Geometry check sheet. Reference: the model listing, model coordinates, mm. Face numbers are marked on the shaded views. A direction names the side the tool comes from. Give positions to 0.01 mm unless a question says otherwise; leave off trailing zeros. Loops run counter-clockwise (first coordinate to the right, second up) from the corner with the lowest first, then second, coordinate; pieces in that order, holes last. Notation, with made-up numbers: (9.25, -38) - (33.25, -38) arc R24 ccw to (33.25, 0) - close; hole circle Ø9 at (-2.5, -36.5). An arc over 180 degrees is marked (long way). Use a Markdown table: item, result. Add a question column.
1. Cross-section at C-C on y = 8.75. Enter the section's corners in (x, z), and give its area (3 significant figures).
2. Draft check along Z on the marked faces 1, 2 and 3. Enter one of: pulls with the +Z half, pulls with the -Z half, needs draft (parallel to the pull), parting line crosses it, or undercut.
3. Set-up check for the marked faces 4, 5, 6, 7 and 8: record each of +Z, -Z, +X, -X, +Y, -Y from which the full face is reachable in a straight line by a thin tool's end or side.
4. Cross-section at B-B on z = 6. Enter the section's corners in (x, y), and give its area (3 significant figures).
5. Cross-section at D-D on x = 15. Enter the section's corners in (y, z).
6. Material ranges on L1, parallel to X at y = 3.65, z = 6; L2, parallel to Z at x = -15, y = 3.85; L3, parallel to X at y = 8.75, z = 8, recorded low to high.
7. Depth check by flat-ended pin: P1, Ø2, axis at y = 7, z = 9, coming from the -X side; P2, Ø3.5, axis at x = 17.5, z = 9, coming from the +Y side; P3, Ø5, axis at x = -1, z = 4.5, coming from the -Y side. Enter the tip coordinate at first touch or a pass-through.
8. Cross-section at A-A on y = 2.75. Enter the section's corners in (x, z).
from build123d import *

# Parameters (mm, degrees)
EXTRUDE_1_DEPTH     = 12
SKETCH_2_R          = 1.9
CUT_EXTRUDE_5_DEPTH = 30.966648128


with BuildPart() as part:
    # 草图1 → 凸台-拉伸1 (new body)
    with BuildSketch(Plane.XY):
        Polygon((-11, 15), (11, 15), (11, 5), (23, 5), (23, 0), (6, 0), (6, 10), (-6, 10), (-6, 0), (-23, 0), (-23, 5), (-11, 5), align=None)
    extrude(amount=EXTRUDE_1_DEPTH)

    # 草图2 → 切除-拉伸5 (cut, through all)
    with BuildSketch(Plane(origin=(0, 0, 0), x_dir=(1, 0, 0), z_dir=(0, 1, 0))):
        with Locations((-15, -6)):
            Circle(SKETCH_2_R)
        with Locations(Location((15, -6, 0), (0, 0, 90))):
            Circle(SKETCH_2_R)
    extrude(amount=CUT_EXTRUDE_5_DEPTH, mode=Mode.SUBTRACT)


solid = part.part
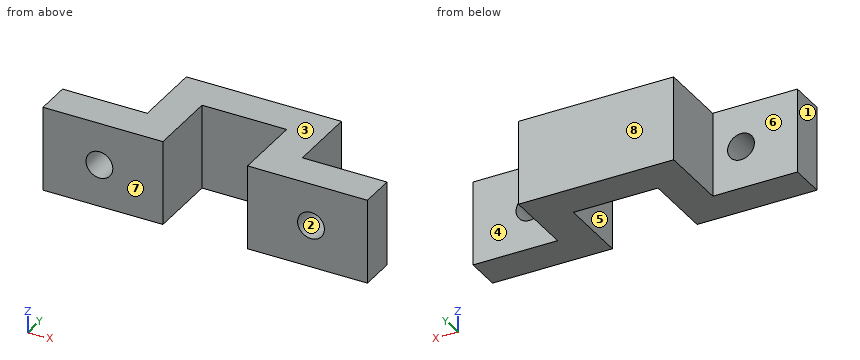
Values found:
| question | item | result |
|---|---|---|
| 1 | outline | (-11, 0) - (-6, 0) - (-6, 12) - (-11, 12) - close; (6, 0) - (11, 0) - (11, 12) - (6, 12) - close |
| 1 | area | 120 mm2 |
| 2 | face 1 | needs draft |
| 2 | face 2 | undercut |
| 2 | face 3 | pulls with the +Z half |
| 3 | face 4 | +Z, -Z, +X, +Y |
| 3 | face 5 | +Z, -Z, -Y |
| 3 | face 6 | +Z, -Z, -X, +Y |
| 3 | face 7 | +Z, -Z, +X, -X, -Y |
| 3 | face 8 | +Z, -Z, +X, -X, +Y |
| 4 | outline | (-23, 0) - (-16.9, 0) - (-16.9, 5) - (-23, 5) - close; (-13.1, 0) - (-6, 0) - (-6, 10) - (6, 10) - (6, 0) - (13.1, 0) - (13.1, 5) - (11, 5) - (11, 15) - (-11, 15) - (-11, 5) - (-13.1, 5) - close; (16.9, 0) - (23, 0) - (23, 5) - (16.9, 5) - close |
| 4 | area | 292 mm2 |
| 5 | outline | (0, 0) - (5, 0) - (5, 4.1) - (0, 4.1) - close; (0, 7.9) - (5, 7.9) - (5, 12) - (0, 12) - close |
| 6 | L1 | x = -23 to -16.9, -13.1 to -6, 6 to 13.1, 16.9 to 23 |
| 6 | L2 | z = 0 to 4.1, 7.9 to 12 |
| 6 | L3 | x = -11 to -6, 6 to 11 |
| 7 | P1 | stops at x = -11 |
| 7 | P2 | stops at y = 5 |
| 7 | P3 | stops at y = 10 |
| 8 | outline | (-23, 0) - (-6, 0) - (-6, 12) - (-23, 12) - close; (6, 0) - (23, 0) - (23, 12) - (6, 12) - close; hole circle Ø3.8 at (-15, 6); hole circle Ø3.8 at (15, 6) |
